from build123d import *

# Parameters (mm, degrees)
F1_DEPTH = 2
F2_DEPTH = 8
F3_DEPTH = 8
F4_DEPTH = 7.25


with BuildPart() as f1:
    # F0 (on Top) → F1 (new body)
    with BuildSketch(Plane.XY):
        with BuildLine():
            Line((4.85, 7.2), (-4.85, 7.2))
            ThreePointArc((-4.85, 7.2), (-6.5117009358, 6.5117009358), (-7.2, 4.85))
            Line((-7.2, 4.85), (-7.2, -4.85))
            ThreePointArc((-7.2, -4.85), (-6.5117009358, -6.5117009358), (-4.85, -7.2))
            Line((-4.85, -7.2), (4.85, -7.2))
            ThreePointArc((4.85, -7.2), (6.5117009358, -6.5117009358), (7.2, -4.85))
            Line((7.2, -4.85), (7.2, 4.85))
            ThreePointArc((7.2, 4.85), (6.5117009358, 6.5117009358), (4.85, 7.2))
        make_face()
        with BuildLine():
            ThreePointArc((6.45, -4.85), (5.9813708499, -5.9813708499), (4.85, -6.45))
            Line((4.85, -6.45), (-4.85, -6.45))
            ThreePointArc((-4.85, -6.45), (-5.9813708499, -5.9813708499), (-6.45, -4.85))
            Line((-6.45, -4.85), (-6.45, 4.85))
            ThreePointArc((-6.45, 4.85), (-5.9813708499, 5.9813708499), (-4.85, 6.45))
            Line((-4.85, 6.45), (4.85, 6.45))
            ThreePointArc((4.85, 6.45), (5.9813708499, 5.9813708499), (6.45, 4.85))
            Line((6.45, 4.85), (6.45, -4.85))
        make_face(mode=Mode.SUBTRACT)
    extrude(amount=F1_DEPTH)

    # F0 (on Top) → F2 (join)
    with BuildSketch(Plane.XY):
        with BuildLine():
            Line((-4.85, -6.45), (4.85, -6.45))
            ThreePointArc((4.85, -6.45), (5.9813708499, -5.9813708499), (6.45, -4.85))
            Line((6.45, -4.85), (6.45, 4.85))
            ThreePointArc((6.45, 4.85), (5.9813708499, 5.9813708499), (4.85, 6.45))
            Line((4.85, 6.45), (-4.85, 6.45))
            ThreePointArc((-4.85, 6.45), (-5.9813708499, 5.9813708499), (-6.45, 4.85))
            Line((-6.45, 4.85), (-6.45, -4.85))
            ThreePointArc((-6.45, -4.85), (-5.9813708499, -5.9813708499), (-4.85, -6.45))
        make_face()
        Polygon((1.063809, -3.535861), (0.026241, -3.535861), (0.026241, -2.115779), (-3.330316, -2.115779), (0.743454, 3.535861), (1.063809, 3.535861), (1.063809, -1.322063), (1.914902, -1.322063), (1.914902, -2.115779), (1.063809, -2.115779), align=None, mode=Mode.SUBTRACT)
    extrude(amount=F2_DEPTH)



with BuildPart() as f3:
    # F0 (on Top) → F3 (new body)
    with BuildSketch(Plane.XY):
        Polygon((0.033413, 0.820014), (0.05493, 1.192964), (-1.72854, -1.322063), (0.026241, -1.322063), (0.026241, 0.499658), align=None)
    extrude(amount=F3_DEPTH)


with BuildPart() as f1_1:
    add(f1.part)

    add(f3.part)  # F4 merges F3
    # F0 (on Top) → F4 (join)
    with BuildSketch(Plane.XY):
        Polygon((0.026241, -2.115779), (0.026241, -3.535861), (1.063809, -3.535861), (1.063809, -2.115779), (1.914902, -2.115779), (1.914902, -1.322063), (1.063809, -1.322063), (1.063809, 3.535861), (0.743454, 3.535861), (-3.330316, -2.115779), align=None)
        Polygon((-1.72854, -1.322063), (0.05493, 1.192964), (0.033413, 0.820014), (0.026241, 0.499658), (0.026241, -1.322063), align=None, mode=Mode.SUBTRACT)
    extrude(amount=F4_DEPTH)


solid = f1_1.part
Input: part model. Units: mm. Frame: model coordinates. A direction names the side the tool comes from. Coordinates: 2 decimals unless noted, no trailing zeros. Loops run counter-clockwise (first coordinate to the right, second up) from the corner with the lowest first, then second, coordinate; pieces in that order, holes last. Notation, with made-up numbers: (-6, 30) - (34, 30) arc R25 cw to (34, 65) - close; hole circle Ø2 at (-6.5, 58.5). An arc over 180 degrees is marked (long way). Answer in a Markdown table with one row per item. Add a question column.
Item 1: Section query D-D on x = -2.5. Return the cut outline in (y, z).
Item 2: Access query for faces 4 (the flat face through (0, -6.45, 5)), 5 (the flat face through (0, 6.45, 5)), 6 (the flat face through (-0.824, -0.047, 7.62)), 7 (the cylindrical face through (5.97, -5.99, 4.96)), 8 (the flat face through (-6.45, 0, 5)). Directions: +Z, -Z, +X, -X, +Y, -Y. A direction counts if a zero-diameter tool reaches every point of the face in a straight line with its end or side. Return the directions, or none.
Item 3: Section query C-C on y = -2.75. Return the cut outline in (x, z).
Item 4: Section query A-A on z = 7.5. Return the cut outline in (x, y).
Item 5: Mould query, pull axis Y, two halves, no side actions, for faces 1 (the flat face through (1.3, 0.1, 8)), 2 (the cylindrical face through (-5.97, 5.99, 4.96)), 3 (the flat face through (-1.3, 0.7, 7.6)). Classes: released by +Y, released by -Y, zero draft, split by the parting line, or undercut.
Item 6: Line query: line 1 along X through (y, z) = (-1.25, 5.5); line 2 along Y through (x, z) = (-5, 1.25). Output: solid intervals per line, ascending. Write a range as [from, to].
Item 7: Contact query for flat-ended pins moving along their axis: P1, Ø1.8, axis at x = 2, z = 4.5, coming from the -Y side; P2, Ø1.8, axis at y = 2, z = 5, coming from the +X side; P3, Ø1.5, axis at x = -0.5, z = 4, coming from the +Y side; P4, Ø5, axis at x = -1.5, y = -1, coming from the -Z side. Output: stop coordinate, or through.
Item 8: Section query B-B on z = 1.25. Return the cut outline in (x, y).
Recorded:
| question | item | result |
|---|---|---|
| 1 | outline | (-7.2, 0) - (7.2, 0) - (7.2, 2) - (6.45, 2) - (6.45, 8) - (-0.96, 8) - (-0.96, 7.25) - (-2.12, 7.25) - (-2.12, 8) - (-6.45, 8) - (-6.45, 2) - (-7.2, 2) - close |
| 2 | face 4 | +Z, +X, -X, -Y |
| 2 | face 5 | +Z, +X, -X, +Y |
| 2 | face 6 | +Z |
| 2 | face 7 | +Z, +X, -Y |
| 2 | face 8 | +Z, -X, +Y, -Y |
| 3 | outline | (-7.2, 0) - (7.2, 0) - (7.2, 2) - (6.45, 2) - (6.45, 8) - (1.06, 8) - (1.06, 7.25) - (0.03, 7.25) - (0.03, 8) - (-6.45, 8) - (-6.45, 2) - (-7.2, 2) - close |
| 4 | outline | (-6.45, -4.85) arc R1.6 ccw to (-4.85, -6.45) - (4.85, -6.45) arc R1.6 ccw to (6.45, -4.85) - (6.45, 4.85) arc R1.6 ccw to (4.85, 6.45) - (-4.85, 6.45) arc R1.6 ccw to (-6.45, 4.85) - close; (-1.73, -1.32) - (0.03, -1.32) - (0.03, 0.5) - (0.03, 0.82) - (0.05, 1.19) - close; hole (-3.33, -2.12) - (0.03, -2.12) - (0.03, -3.54) - (1.06, -3.54) - (1.06, -2.12) - (1.91, -2.12) - (1.91, -1.32) - (1.06, -1.32) - (1.06, 3.54) - (0.74, 3.54) - close |
| 5 | face 1 | zero draft |
| 5 | face 2 | released by +Y |
| 5 | face 3 | undercut |
| 6 | line 1 | [-6.45, 6.45] |
| 6 | line 2 | [-7.2, 7.2] |
| 7 | P1 | y = -6.45 |
| 7 | P2 | x = 6.45 |
| 7 | P3 | y = 6.45 |
| 7 | P4 | z = 0 |
| 8 | outline | (-7.2, -4.85) arc R2.35 ccw to (-4.85, -7.2) - (4.85, -7.2) arc R2.35 ccw to (7.2, -4.85) - (7.2, 4.85) arc R2.35 ccw to (4.85, 7.2) - (-4.85, 7.2) arc R2.35 ccw to (-7.2, 4.85) - close |
